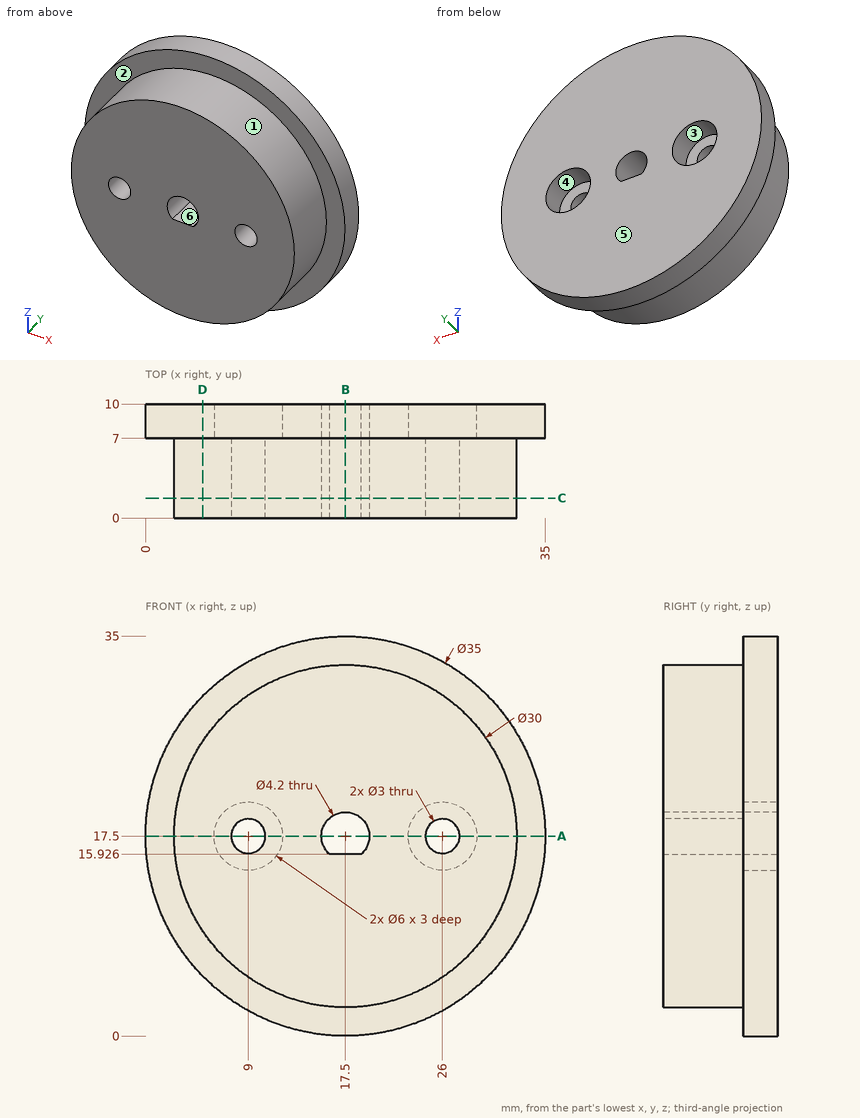
The figure shows three views and two pictorial views of one solid part (mm, origin at its lowest corner). Answer the questions. A direction names the side the tool comes from. Round coordinates to 2 decimals unless told otherwise and drop trailing zeros. Write each loop counter-clockwise with the first axis right and the second up, starting at its lowest first coordinate (ties: lowest second). Pieces come first, ordered by that corner, then holes. Notation, with made-up numbers: (58.5, -18) -> (113.5, -18) arc R20 ccw to (113.5, 18) -> close; hole circle Ø2 at (54.5, 35). An arc over 180 degrees is marked (long way). Answer as a JSON object with one key per item and string values. Group by question number.
Q1. Each of these flat-tipped pins is pushed along its axis until it touches: pin 1 Ø2 at (y, z) = (8, 25) entering from -X; pin 2 Ø3 at (x, z) = (8, 18) entering from +Y; pin 3 Ø6 at (x, y) = (15.5, 2) entering from +Z. Where does it stop, or does it pass through?
Q2. Section C-C (y = 1.75) is taken. Write down the section's boundary in (x, z), plus the area to 3 significant figures.
Q3. Determine the mould class of the marked faces 1, 2 and 3 for opening direction X: pulls with the +X half, pulls with the -X half, needs draft (parallel to the pull), parting line crosses it, or undercut.
Q4. Section D-D (x = 5) is taken. Write down the section's boundary in (y, z).
Q5. Section A-A (z = 17.5) is taken. Write down the section's boundary in (x, y), plus the area to 3 significant figures.
Q6. Straight lines are drawn through the part: line 1 along Z through (x, y) = (9, 8.75); line 2 along Z through (x, y) = (8.5, 9.5); line 3 along Y through (x, z) = (31, 24.5). For each, find the intervals that lie inside material, in ascending order.
Q7. Section B-B (x = 17.5) is taken. Write down the section's boundary in (y, z).
Q8. Which of the six approach directions +Z, -Z, +X, -X, +Y, -Y give full straight-line access (tool end or side, diameter ignored) to the marked faces 4, 5 and 6?
Check values:
{
 "1": {"pin 1": "x = 1.25", "pin 2": "y = 7", "pin 3": "z = 32.5"},
 "2": {"outline": "circle Ø30 at (17.5, 17.5); hole circle Ø3 at (9, 17.5); hole (16.11, 15.93) -> (18.89, 15.93) arc R2.1 ccw (long way) to start; hole circle Ø3 at (26, 17.5)", "area": "680 mm^2"},
 "3": {"face 1": "parting line crosses it", "face 2": "needs draft", "face 3": "undercut"},
 "4": {"outline": "(0, 9.21) -> (7, 9.21) -> (7, 5.25) -> (10, 5.25) -> (10, 29.75) -> (7, 29.75) -> (7, 25.79) -> (0, 25.79) -> close"},
 "5": {"outline": "(0, 7) -> (2.5, 7) -> (2.5, 0) -> (7.5, 0) -> (7.5, 7) -> (6, 7) -> (6, 10) -> (0, 10) -> close; (10.5, 0) -> (15.4, 0) -> (15.4, 10) -> (12, 10) -> (12, 7) -> (10.5, 7) -> close; (19.6, 0) -> (24.5, 0) -> (24.5, 7) -> (23, 7) -> (23, 10) -> (19.6, 10) -> close; (27.5, 0) -> (32.5, 0) -> (32.5, 7) -> (35, 7) -> (35, 10) -> (29, 10) -> (29, 7) -> (27.5, 7) -> close", "area": "195 mm^2"},
 "6": {"line 1": "2.2 to 14.5, 20.5 to 32.8", "line 2": "2.49 to 14.54, 20.46 to 32.51", "line 3": "7 to 10"},
 "7": {"outline": "(0, 2.5) -> (7, 2.5) -> (7, 0) -> (10, 0) -> (10, 15.93) -> (0, 15.93) -> close; (0, 19.6) -> (10, 19.6) -> (10, 35) -> (7, 35) -> (7, 32.5) -> (0, 32.5) -> close"},
 "8": {"face 4": "+Y", "face 5": "+Z, -Z, +X, -X, +Y", "face 6": "+Y, -Y"}
}
